The listing builds one solid part. Answer for the finished solid, in the listing's coordinates (mm). A direction names the side the tool comes from. Give positions to 0.01 mm unless a question says otherwise; leave off trailing zeros. Write each loop counter-clockwise with the first axis right and the second up, starting at its lowest first coordinate (ties: lowest second). Pieces come first, ordered by that corner, then holes. Notation, with made-up numbers: (67.25, 88.25) - (119.25, 88.25) arc R18 cw to (119.25, 97.25) - close; hole circle Ø8 at (67, -13). An arc over 180 degrees is marked (long way). Return JSON: item names as keys, results as strings.
from build123d import *

# Parameters (mm, degrees)
SKETCH_2_R          = 1.5
SKETCH_2_R_2        = 1.55
SKETCH_2_W          = 58.95
SKETCH_2_H          = 34.26
SKETCH_2_W_2        = 25.458045559
SKETCH_2_H_2        = 37.682827862
SKETCH_2_W_3        = 52.836453453
SKETCH_2_H_3        = 38.433812924
EXTRUDE_2_DEPTH     = 3
FILLET_2_R          = 3
FILLET_3_R          = 5
CUT_EXTRUDE_1_DEPTH = 157.537629335


with BuildPart() as part:
    # 草图2 → 凸台-拉伸2 (new body)
    with BuildSketch(Plane(origin=(0, 0, 0), x_dir=(1, 0, 0), z_dir=(0, 1, 0))):
        with BuildLine():
            Line((-72.5, -36.293945631), (-72.5, -107.5))
            ThreePointArc((-72.5, -107.5), (-69.571067812, -114.571067812), (-62.5, -117.5))
            Line((-62.5, -117.5), (93.386553273, -117.5))
            ThreePointArc((93.386553273, -117.5), (100.457621085, -114.571067812), (103.386553273, -107.5))
            Line((103.386553273, -107.5), (103.386553273, 107.5))
            ThreePointArc((103.386553273, 107.5), (100.457621085, 114.571067812), (93.386553273, 117.5))
            Line((93.386553273, 117.5), (-62.5, 117.5))
            ThreePointArc((-62.5, 117.5), (-69.571067812, 114.571067812), (-72.5, 107.5))
            Line((-72.5, 107.5), (-72.5, 36.293945631))
            Line((-72.5, 36.293945631), (-40.778460838, 36.293945631))
            Line((-40.778460838, 36.293945631), (-40.778460838, -36.293945631))
            Line((-40.778460838, -36.293945631), (-72.5, -36.293945631))
        make_face()
        with Locations(Location((-35, 35, 0), (0, 0, 270))):
            Circle(SKETCH_2_R, mode=Mode.SUBTRACT)
        with Locations(Location((35, 35, 0), (0, 0, 90))):
            Circle(SKETCH_2_R, mode=Mode.SUBTRACT)
        with Locations(Location((35, -35, 0), (0, 0, 270))):
            Circle(SKETCH_2_R, mode=Mode.SUBTRACT)
        with Locations(Location((-35, -35, 0), (0, 0, 90))):
            Circle(SKETCH_2_R, mode=Mode.SUBTRACT)
        with Locations(Location((-17.5, 35, 0), (0, 0, 270))):
            Circle(SKETCH_2_R, mode=Mode.SUBTRACT)
        with Locations(Location((17.5, 35, 0), (0, 0, 90))):
            Circle(SKETCH_2_R, mode=Mode.SUBTRACT)
        with Locations(Location((-17.5, -35, 0), (0, 0, 90))):
            Circle(SKETCH_2_R, mode=Mode.SUBTRACT)
        with Locations(Location((17.5, -35, 0), (0, 0, 270))):
            Circle(SKETCH_2_R, mode=Mode.SUBTRACT)
        with Locations(Location((-35, 17.5, 0), (0, 0, 270))):
            Circle(SKETCH_2_R, mode=Mode.SUBTRACT)
        with Locations(Location((-35, -17.5, 0), (0, 0, 90))):
            Circle(SKETCH_2_R, mode=Mode.SUBTRACT)
        with Locations(Location((35, -17.5, 0), (0, 0, 270))):
            Circle(SKETCH_2_R, mode=Mode.SUBTRACT)
        with Locations(Location((35, 17.5, 0), (0, 0, 90))):
            Circle(SKETCH_2_R, mode=Mode.SUBTRACT)
        with Locations(Location((0, 35, 0), (0, 0, 270))):
            Circle(SKETCH_2_R, mode=Mode.SUBTRACT)
        with Locations(Location((0, -35, 0), (0, 0, 270))):
            Circle(SKETCH_2_R, mode=Mode.SUBTRACT)
        with Locations(Location((-49.509707517, -52.404109444, 0), (0, 0, 270))):
            Circle(SKETCH_2_R, mode=Mode.SUBTRACT)
        with Locations(Location((-49.509707517, -96.664109444, 0), (0, 0, 270))):
            Circle(SKETCH_2_R, mode=Mode.SUBTRACT)
        with Locations(Location((19.440292483, -52.404109444, 0), (0, 0, 270))):
            Circle(SKETCH_2_R, mode=Mode.SUBTRACT)
        with Locations(Location((19.440292483, -96.664109444, 0), (0, 0, 270))):
            Circle(SKETCH_2_R, mode=Mode.SUBTRACT)
        with Locations(Location((-59.25, -76.75, 0), (0, 0, 270))):
            Circle(SKETCH_2_R, mode=Mode.SUBTRACT)
        with Locations(Location((79.75, -76.75, 0), (0, 0, 270))):
            Circle(SKETCH_2_R, mode=Mode.SUBTRACT)
        with Locations(Location((79.75, 76.75, 0), (0, 0, 270))):
            Circle(SKETCH_2_R, mode=Mode.SUBTRACT)
        with Locations(Location((-59.25, 76.75, 0), (0, 0, 270))):
            Circle(SKETCH_2_R, mode=Mode.SUBTRACT)
        with Locations(Location((-68.87108956, 94.711076741, 0), (0, 0, 270))):
            Circle(SKETCH_2_R, mode=Mode.SUBTRACT)
        with Locations(Location((-68.87108956, 47.711076741, 0), (0, 0, 270))):
            Circle(SKETCH_2_R, mode=Mode.SUBTRACT)
        with Locations(Location((9.12891044, 47.711076741, 0), (0, 0, 270))):
            Circle(SKETCH_2_R, mode=Mode.SUBTRACT)
        with Locations(Location((9.12891044, 94.711076741, 0), (0, 0, 270))):
            Circle(SKETCH_2_R, mode=Mode.SUBTRACT)
        with Locations(Location((48.531405595, -36.854109444, 0), (0, 0, 270))):
            Circle(SKETCH_2_R_2, mode=Mode.SUBTRACT)
        with Locations(Location((84.091405595, -36.854109444, 0), (0, 0, 270))):
            Circle(SKETCH_2_R_2, mode=Mode.SUBTRACT)
        with Locations(Location((48.531405595, -98.234109444, 0), (0, 0, 270))):
            Circle(SKETCH_2_R_2, mode=Mode.SUBTRACT)
        with Locations(Location((84.091405595, -98.234109444, 0), (0, 0, 270))):
            Circle(SKETCH_2_R_2, mode=Mode.SUBTRACT)
        with Locations(Location((46.131405595, 37.969626598, 0), (0, 0, 270))):
            Circle(SKETCH_2_R, mode=Mode.SUBTRACT)
        with Locations(Location((83.131405595, 37.969626598, 0), (0, 0, 270))):
            Circle(SKETCH_2_R, mode=Mode.SUBTRACT)
        with Locations(Location((46.131405595, -24.030373402, 0), (0, 0, 270))):
            Circle(SKETCH_2_R, mode=Mode.SUBTRACT)
        with Locations(Location((83.131405595, -24.030373402, 0), (0, 0, 270))):
            Circle(SKETCH_2_R, mode=Mode.SUBTRACT)
        with BuildLine():
            Line((-18.1, 22.5), (18.1, 22.5))
            ThreePointArc((18.1, 22.5), (21.211269837, 21.211269837), (22.5, 18.1))
            Line((22.5, 18.1), (22.5, -18.1))
            ThreePointArc((22.5, -18.1), (21.211269837, -21.211269837), (18.1, -22.5))
            Line((18.1, -22.5), (-18.1, -22.5))
            ThreePointArc((-18.1, -22.5), (-21.211269837, -21.211269837), (-22.5, -18.1))
            Line((-22.5, -18.1), (-22.5, 18.1))
            ThreePointArc((-22.5, 18.1), (-21.211269837, 21.211269837), (-18.1, 22.5))
        make_face(mode=Mode.SUBTRACT)
        with Locations((-15.034707517, -74.534109444)):
            Rectangle(SKETCH_2_W, SKETCH_2_H, mode=Mode.SUBTRACT)
        with Locations((75.885013297, 0)):
            Rectangle(SKETCH_2_W_2, SKETCH_2_H_2, mode=Mode.SUBTRACT)
        with Locations((-23.799399193, 71.645143509)):
            Rectangle(SKETCH_2_W_3, SKETCH_2_H_3, mode=Mode.SUBTRACT)
    extrude(amount=EXTRUDE_2_DEPTH)

    # 圆角2
    fillet_2_edges = [part.edges().sort_by_distance(p)[0] for p in [
        (-72.5, 1.5, 36.293945631),
        (-40.778460838, 1.5, 36.293945631),
        (-40.778460838, 1.5, -36.293945631),
        (-72.5, 1.5, -36.293945631),
    ]]
    fillet(fillet_2_edges, radius=FILLET_2_R)

    # 圆角3
    fillet_3_edges = [part.edges().sort_by_distance(p)[0] for p in [
        (88.614036076, 1.5, 18.841413931),
        (88.614036076, 1.5, -18.841413931),
        (63.155990517, 1.5, -18.841413931),
        (63.155990517, 1.5, 18.841413931),
    ]]
    fillet(fillet_3_edges, radius=FILLET_3_R)

    # 草图3 → 切除-拉伸1 (cut, through all)
    with BuildSketch(Plane(origin=(0, 3, 0), x_dir=(1, 0, 0), z_dir=(0, 1, 0))):
        with BuildLine():
            Line((30.380318315, 106.392706566), (66.1383582, 106.392706566))
            ThreePointArc((66.1383582, 106.392706566), (73.287559025, 99.243505741), (66.1383582, 92.094304917))
            Line((66.1383582, 92.094304917), (30.380318315, 92.094304917))
            ThreePointArc((30.380318315, 92.094304917), (23.23111749, 99.243505741), (30.380318315, 106.392706566))
        make_face()
        with BuildLine():
            Line((30.380318315, 62.274503657), (66.1383582, 62.274503657))
            ThreePointArc((66.1383582, 62.274503657), (72.736553362, 55.676308496), (66.1383582, 49.078113334))
            Line((66.1383582, 49.078113334), (30.380318315, 49.078113334))
            ThreePointArc((30.380318315, 49.078113334), (23.782123153, 55.676308496), (30.380318315, 62.274503657))
        make_face()
    extrude(amount=-CUT_EXTRUDE_1_DEPTH, mode=Mode.SUBTRACT)


solid = part.part
Item 1: A cutting plane is placed at A-A on z = -100. Determine the outline of the cut face in (x, y).
Answer below:
{"outline": "(-72.5, 0) - (23.27, 0) - (23.27, 3) - (-72.5, 3) - close; (73.25, 0) - (103.39, 0) - (103.39, 3) - (73.25, 3) - close"}
Item 2: Flat-ended cylindrical pins translate along their axes: P1, Ø2.5, axis at x = -17.5, z = -35, coming from the -Y side; P2, Ø1.5, axis at y = 2, z = 12.5, coming from the -X side. Find the tip coordinate at first contact, or state that the pin passes through.
Answer below:
{"P1": "passes through", "P2": "stops at x = -40.78"}
Item 3: Consider L1, parallel to Z at x = -11.5, y = 0.8; L2, parallel to Z at x = -45.5, y = 2.1; L3, parallel to Z at x = 39.5, y = 0.4. Determine where each line is inside the solid, lowest interval first.
Answer below:
{"L1": "z = -117.5 to -90.86, -52.43 to -22.5, 22.5 to 57.4, 91.66 to 117.5", "L2": "z = -117.5 to -90.86, -52.43 to -36.29, 36.29 to 117.5", "L3": "z = -117.5 to -106.39, -92.09 to -62.27, -49.08 to 117.5"}
Item 4: The mould has two halves that part along Z. Classify faces 1 (the face through (87.188, 1.521, -17.338)), 2 (the face through (34, 0, -2)), 3 (the face through (64.582, 1.521, -17.338)), 4 (the face through (100.535, 1.479, -114.493)): +Z half, -Z half, draft (parallel to the pull), parting line (faces both ways), or undercut.
Answer below:
{"face 1": "undercut", "face 2": "draft", "face 3": "undercut", "face 4": "-Z half"}
Item 5: A cutting plane is placed at B-B on y = 1.5. Give the number of separate pieces and of enclosed holes in the cut face, then the cut area to 3 significant figures.
Answer below:
{"separate pieces": "1", "enclosed holes": "40", "area": "30,400 mm²"}
Item 6: For faces 5 (the face through (73.286, 1.521, -99.401)), 6 (the face through (-69.49, 1.48, -114.65)), determine the directions among +Z, -Z, +X, -X, +Y, -Y from which every point of the face is accessible in a straight line to the end or side of a thin tool.
Answer below:
{"face 5": "+Y, -Y", "face 6": "-Z, -X, +Y, -Y"}
